The model under review builds one solid part; all positions refer to its coordinate system, in mm. Face numbers are marked on the shaded views. A direction names the side the tool comes from. Round coordinates to 2 decimals unless told otherwise and drop trailing zeros. Order: outer loops, then holes, each group sorted by start corner. A loop starts at its lowest first (then second) coordinate and runs counter-clockwise, first axis right, second up.
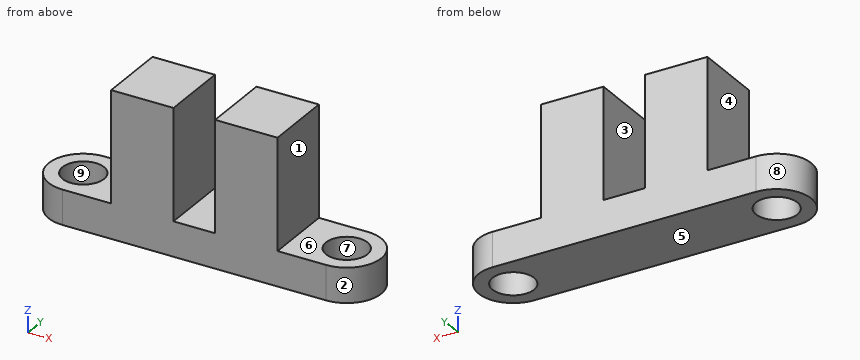
```python
from build123d import *

# Parameters (mm, degrees)
SKETCH_1_R      = 1.5
EXTRUDE_1_DEPTH = 2.5
SKETCH_2_W      = 4.5
SKETCH_2_H      = 5
EXTRUDE_2_DEPTH = 8


with BuildPart() as part:
    # ｽｹｯﾁ1 → ﾎﾞｽ - 押し出し1 (new body)
    with BuildSketch(Plane.XY):
        with BuildLine():
            Line((0, 2.5), (19, 2.5))
            ThreePointArc((19, 2.5), (21.5, 0), (19, -2.5))
            Line((19, -2.5), (0, -2.5))
            ThreePointArc((0, -2.5), (-2.5, 0), (0, 2.5))
        make_face()
        Circle(SKETCH_1_R, mode=Mode.SUBTRACT)
        with Locations((19, 0)):
            Circle(SKETCH_1_R, mode=Mode.SUBTRACT)
    extrude(amount=EXTRUDE_1_DEPTH)

    # ｽｹｯﾁ2 → ﾎﾞｽ - 押し出し2 (add)
    with BuildSketch(Plane.XY.offset(2.5)):
        with Locations((5.75, 0)):
            Rectangle(SKETCH_2_W, SKETCH_2_H)
        with Locations((13.25, 0)):
            Rectangle(SKETCH_2_W, SKETCH_2_H)
    extrude(amount=EXTRUDE_2_DEPTH)


solid = part.part
```
(1) Consider section C-C (z = 2). Write out the cut boundary in (x, y).
Data:
outline: (0, -2.5) - (19, -2.5) arc R2.5 ccw to (19, 2.5) - (0, 2.5) arc R2.5 ccw to start; hole circle Ø3 at (0, 0); hole circle Ø3 at (19, 0)
(2) Consider section D-D (y = 1.75). Write out the cut boundary in (x, z), and give its area (3 significant figures).
Data:
outline: (-1.79, 0) - (20.79, 0) - (20.79, 2.5) - (15.5, 2.5) - (15.5, 10.5) - (11, 10.5) - (11, 2.5) - (8, 2.5) - (8, 10.5) - (3.5, 10.5) - (3.5, 2.5) - (-1.79, 2.5) - close
area: 128 mm2
(3) To check wall thickness, follow probe 1 along Y at (x, z) = (0, 1.1); probe 2 along X at (y, z) = (0.1, 6.25); probe 3 along Z at (x, y) = (17.5, 1.2). State the ranges of each line that lie inside material, in increasing order.
Data:
probe 1: y = -2.5 to -1.5, 1.5 to 2.5
probe 2: x = 3.5 to 8, 11 to 15.5
probe 3: z = 0 to 2.5
(4) Consider section A-A (z = 7.5). Write out the cut boundary in (x, y), and give its area (3 significant figures).
Data:
outline: (3.5, -2.5) - (8, -2.5) - (8, 2.5) - (3.5, 2.5) - close; (11, -2.5) - (15.5, -2.5) - (15.5, 2.5) - (11, 2.5) - close
area: 45.0 mm2
(5) Draft analysis for pull direction Y (two halves, no side actions). For the marked faces 6, 7, 8 and 9, state which applies: pulls with the +Y half, pulls with the -Y half, needs draft (parallel to the pull), parting line crosses it, or undercut.
Data:
face 6: needs draft
face 7: undercut
face 8: parting line crosses it
face 9: undercut
(6) For the marked faces 1, 2, 3, 4 and 5, list the 3-axis set-ups (+Z, -Z, +X, -X, +Y, -Y) from which the entire face can be reached by the end or side of a thin tool; tool diameter is ignored.
Data:
face 1: +Z, +X, +Y, -Y
face 2: +Z, -Z, +X
face 3: +Z, +Y, -Y
face 4: +Z, -X, +Y, -Y
face 5: -Z, +X, -X, +Y, -Y
(7) Insertion check: pin 1 (1.5 mm diameter, centred on y = -0.5, z = 4, fed in from -X); pin 2 (2.5 mm diameter, centred on y = 0.5, z = 4.5, fed in from +X); pin 3 (2.5 mm diameter, centred on x = 9.5, y = 1, fed in from +Z). Each pin has a flat end and moves straight along its axis. Give the tip position at first contact, or say it passes through.
Data:
pin 1: stops at x = 3.5
pin 2: stops at x = 15.5
pin 3: stops at z = 2.5
(8) Consider section B-B (y = 0). Write out the cut boundary in (x, z), and give its area (3 significant figures).
Data:
outline: (-2.5, 0) - (-1.5, 0) - (-1.5, 2.5) - (-2.5, 2.5) - close; (1.5, 0) - (17.5, 0) - (17.5, 2.5) - (15.5, 2.5) - (15.5, 10.5) - (11, 10.5) - (11, 2.5) - (8, 2.5) - (8, 10.5) - (3.5, 10.5) - (3.5, 2.5) - (1.5, 2.5) - close; (20.5, 0) - (21.5, 0) - (21.5, 2.5) - (20.5, 2.5) - close
area: 117 mm2
